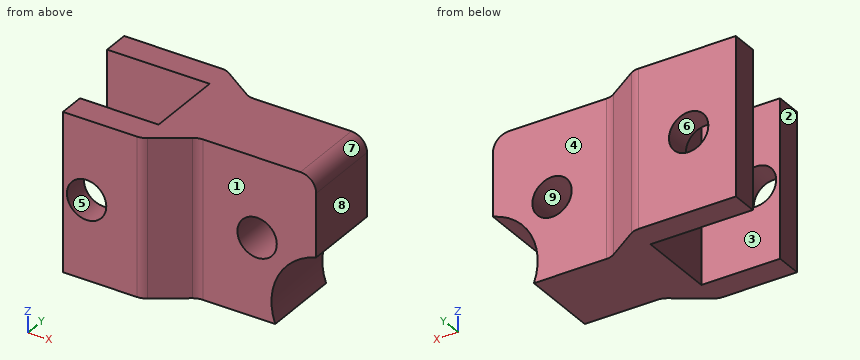
```python
from build123d import *

# Parameters (mm, degrees)
SKETCH1_W               = 12.7
SKETCH1_H               = 4.23164
SKETCH1_W_2             = 16.51
BOSS_EXTRUDE1_DEPTH     = 25.4
CUT_EXTRUDE4_DEPTH      = 49.820594354
CUT_EXTRUDE4_DEPTH_BACK = 49.820594354
SKETCH4_R               = 3.175
CUT_EXTRUDE5_DEPTH      = 49.820594354
CUT_EXTRUDE5_DEPTH_BACK = 49.820594354
SKETCH6_R               = 3.175
CUT_EXTRUDE6_DEPTH      = 49.820594354
CUT_EXTRUDE6_DEPTH_BACK = 49.820594354
FILLET1_R               = 2.54


with BuildPart() as part:
    # Sketch1 → Boss-Extrude1 (new body)
    with BuildSketch(Plane.XY):
        with Locations((6.35, -2.11582)):
            Rectangle(SKETCH1_W, SKETCH1_H)
        Polygon((19.05, 0), (38.1, 0), (38.1, 12.7), (19.05, 12.7), (12.7, 16.93164), (12.7, 12.7), (12.7, 0), (12.7, -4.23164), align=None)
        with Locations((4.445, 14.81582)):
            Rectangle(SKETCH1_W_2, SKETCH1_H)
    extrude(amount=BOSS_EXTRUDE1_DEPTH)

    # Sketch4 → Cut-Extrude4 (cut, two sides: drawn at the far end of the back side and taken through both)
    with BuildSketch(Plane(origin=(0, 0, 0), x_dir=(1, 0, 0), z_dir=(0, 1, 0)).offset(-CUT_EXTRUDE4_DEPTH_BACK)):
        with Locations(Location((3.81, -12.7, 0), (0, 0, 270))):
            Circle(SKETCH4_R)
    extrude(amount=CUT_EXTRUDE4_DEPTH + CUT_EXTRUDE4_DEPTH_BACK, mode=Mode.SUBTRACT)

    # Sketch6 → Cut-Extrude5 (cut, two sides: drawn at the far end of the back side and taken through both)
    with BuildSketch(Plane(origin=(0, 12.7, 0), x_dir=(1, 0, 0), z_dir=(0, 1, 0)).offset(-CUT_EXTRUDE5_DEPTH_BACK)):
        with Locations(Location((28.575, -12.7, 0), (0, 0, 270))):
            Circle(SKETCH6_R)
    extrude(amount=CUT_EXTRUDE5_DEPTH + CUT_EXTRUDE5_DEPTH_BACK, mode=Mode.SUBTRACT)

    # Sketch7 → Cut-Extrude6 (cut, two sides: drawn at the far end of the back side and taken through both)
    with BuildSketch(Plane(origin=(0, 12.7, 0), x_dir=(1, 0, 0), z_dir=(0, 1, 0)).offset(-CUT_EXTRUDE6_DEPTH_BACK)):
        with BuildLine():
            Line((31.497009702, 0), (38.1, 0))
            Line((38.1, 0), (38.1, -12.7))
            ThreePointArc((38.1, -12.7), (31.974019773, -7.818507683), (31.497009702, 0))
        make_face()
    extrude(amount=CUT_EXTRUDE6_DEPTH + CUT_EXTRUDE6_DEPTH_BACK, mode=Mode.SUBTRACT)

    # Fillet1
    fillet1_edges = [part.edges().sort_by_distance(p)[0] for p in [
        (12.7, 16.93164, 12.7),
        (19.05, 12.7, 12.7),
        (19.05, 0, 12.7),
        (12.7, -4.23164, 12.7),
        (38.1, 6.35, 25.4),
    ]]
    fillet(fillet1_edges, radius=FILLET1_R)


solid = part.part
```
Build history of the part. All positions in model axes, mm. Face numbers are marked on the shaded views. A direction names the side the tool comes from. Round coordinates to 2 decimals unless told otherwise and drop trailing zeros. Write each loop counter-clockwise with the first axis right and the second up, starting at its lowest first coordinate (ties: lowest second). Pieces come first, ordered by that corner, then holes.
1) Band-saw the part on B-B, the plane z = 12.25. List the corners of the cut face in (x, y).
2) Band-saw the part on D-D, the plane x = 27. List the corners of the cut face in (y, z).
3) Pin check, flat tips, straight feed: pin 1 (1.5 mm diameter, centred on x = 27, y = 14, fed in from -Z); pin 2 (1.3 mm diameter, centred on y = -3, z = 12, fed in from -X); pin 3 (8 mm diameter, centred on y = 8, z = 6, fed in from +X); pin 4 (14.5 mm diameter, centred on x = 31, z = 18.5, fed in from -Y). Stop position of each tip, or through.
4) Band-saw the part on C-C, the plane y = 0.5. List the corners of the cut face in (x, z) (3 decimals), and give its area (3 significant figures).
5) Drill centre lines: probe 1 along Z at (x, y) = (3.81, -2.2) (3 decimals); probe 2 along Y at (x, z) = (6.5, 7.25); probe 3 along X at (y, z) = (1.5, 13.5). Where is each one in solid material? Low to high.
6) Band-saw the part on A-A, the plane x = 3.81. List the corners of the cut face in (y, z) (3 decimals).
7) 3-axis set-ups, long thin cutter, end or side, ignore diameter. For the marked faces 1, 2, 3, 4 and 5: which of +Z, -Z, +X, -X, +Y, -Y reach the whole face in a straight line?
8) Mould opens along Z. For the marked faces 6, 7, 8 and 9 say: +Z half, -Z half, draft (parallel to the pull), parting line (faces both ways), or undercut.
Ans:
1. outline: (-3.81, 12.7) - (0.67, 12.7) - (0.67, 16.93) - (-3.81, 16.93) - close; (0, -4.23) - (0.67, -4.23) - (0.67, 0) - (0, 0) - close; (6.95, -4.23) - (11.93, -4.23) arc R2.54 ccw to (13.34, -3.81) - (18.41, -0.43) arc R2.54 cw to (19.82, 0) - (25.43, 0) - (25.43, 12.7) - (19.82, 12.7) arc R2.54 cw to (18.41, 13.13) - (13.34, 16.51) arc R2.54 ccw to (11.93, 16.93) - (6.95, 16.93) - (6.95, 12.7) - (12.7, 12.7) - (12.7, 0) - (6.95, 0) - close; (31.72, 0) - (36.77, 0) - (36.77, 12.7) - (31.72, 12.7) - close
2. outline: (0, 0) - (12.7, 0) - (12.7, 9.94) - (0, 9.94) - close; (0, 15.46) - (12.7, 15.46) - (12.7, 25.4) - (0, 25.4) - close
3. pin 1: passes through
3. pin 2: stops at x = 0
3. pin 3: stops at x = 33.53
3. pin 4: stops at y = 0
4. outline: (12.7, 0) - (31.497, 0) arc R9.637 cw to (38.1, 12.7) - (38.1, 22.86) arc R2.54 ccw to (35.56, 25.4) - (12.7, 25.4) - close; hole circle Ø6.35 at (28.575, 12.7)
4. area: 539 mm2
5. probe 1: z = 0 to 9.525, 15.875 to 25.4
5. probe 2: y = -4.23 to 0, 12.7 to 16.93
5. probe 3: x = 12.7 to 25.5, 31.65 to 38.1
6. outline: (-4.232, 0) - (0, 0) - (0, 9.525) - (-4.232, 9.525) - close; (-4.232, 15.875) - (0, 15.875) - (0, 25.4) - (-4.232, 25.4) - close; (12.7, 0) - (16.932, 0) - (16.932, 9.525) - (12.7, 9.525) - close; (12.7, 15.875) - (16.932, 15.875) - (16.932, 25.4) - (12.7, 25.4) - close
7. face 1: +Z, -Z, +X, -Y
7. face 2: +Z, -Z, -X, -Y
7. face 3: +Z, -Z, -X
7. face 4: +Z, -Z, +X, +Y
7. face 5: +Y, -Y
8. face 6: undercut
8. face 7: +Z half
8. face 8: draft
8. face 9: undercut
